from build123d import *

# Parameters (mm, degrees)
ESBO_O1_W                 = 105
ESBO_O1_H                 = 60
RESSALTO_EXTRUS_O1_DEPTH  = 1.7
ESBO_O2_W                 = 60
ESBO_O2_H                 = 15
ESBO_O2_W_2               = 40
RESSALTO_EXTRUS_O2_DEPTH  = 13.6
RESSALTO_EXTRUS_O6_START  = 11.6
ESBO_O3_W                 = 100
ESBO_O3_H                 = 53
RESSALTO_EXTRUS_O6_DEPTH  = 1.5
ESBO_O4_W                 = 62.184169383
ESBO_O4_H                 = 2.54
ESBO_O4_W_2               = 5.08
ESBO_O4_H_2               = 42.957805244
ESBO_O4_W_3               = 56.07185462
RESSALTO_EXTRUS_O8_DEPTH  = 11.6
ESBO_O6_W                 = 21
ESBO_O6_H                 = 22
RESSALTO_EXTRUS_O9_DEPTH  = 16
ESBO_O7_W                 = 25.746964405
ESBO_O7_H                 = 12
RESSALTO_EXTRUS_O10_DEPTH = 10
ESBO_O8_R                 = 1.5
CORTE_EXTRUS_O1_DEPTH     = 31.8
RESSALTO_EXTRUS_O11_DEPTH = 56.905179
CORTE_EXTRUS_O2_DEPTH     = 11
RESSALTO_EXTRUS_O12_START = 1
ESBO_O12_W                = 7
ESBO_O12_H                = 7
RESSALTO_EXTRUS_O12_DEPTH = 4


with BuildPart() as part:
    # Esbo_o1 → Ressalto-extrus_o1 (new body)
    with BuildSketch(Plane.XY):
        Rectangle(ESBO_O1_W, ESBO_O1_H)
    extrude(amount=RESSALTO_EXTRUS_O1_DEPTH)

    # Esbo_o2 → Ressalto-extrus_o2 (add)
    with BuildSketch(Plane.XY.offset(1.7)):
        with Locations((13.2, -12.2)):
            Rectangle(ESBO_O2_W, ESBO_O2_H)
        with Locations((3.2, 10.2)):
            Rectangle(ESBO_O2_W_2, ESBO_O2_H)
    extrude(amount=RESSALTO_EXTRUS_O2_DEPTH)



with BuildPart() as body_2:
    # Esbo_o3 → Ressalto-extrus_o6 (new body)
    with BuildSketch(Plane(origin=(0, 0, 0), x_dir=(-1, 0, 0), z_dir=(0, 0, -1)).offset(RESSALTO_EXTRUS_O6_START)):
        with Locations((2.5, 4.4)):
            Rectangle(ESBO_O3_W, ESBO_O3_H)
    extrude(amount=RESSALTO_EXTRUS_O6_DEPTH)


with BuildPart() as part_1:
    add(part.part)

    add(body_2.part)  # Ressalto-extrus_o8 merges body 2
    # Esbo_o4 → Ressalto-extrus_o8 (add)
    with BuildSketch(Plane.XY.offset(-11.6)):
        with Locations((7.150543675, 26.719832293)):
            Rectangle(ESBO_O4_W, ESBO_O4_H)
        with Locations((45.784919315, 5.42627648)):
            Rectangle(ESBO_O4_W_2, ESBO_O4_H_2)
        with Locations((10.206701056, -18.689881399)):
            Rectangle(ESBO_O4_W_3, ESBO_O4_H)
    extrude(amount=RESSALTO_EXTRUS_O8_DEPTH)

    # Esbo_o6 → Ressalto-extrus_o9 (add)
    with BuildSketch(Plane.XY.offset(1.7)):
        with Locations((-54, -9.6)):
            Rectangle(ESBO_O6_W, ESBO_O6_H)
    extrude(amount=RESSALTO_EXTRUS_O9_DEPTH)

    # Esbo_o7 → Ressalto-extrus_o10 (add)
    with BuildSketch(Plane.XY.offset(-11.6)):
        with Locations((-47.626517798, 17.9)):
            Rectangle(ESBO_O7_W, ESBO_O7_H)
    extrude(amount=RESSALTO_EXTRUS_O10_DEPTH)

    # Esbo_o8 → Corte-extrus_o1 (cut, through all)
    with BuildSketch(Plane(origin=(0, 0, -13.1), x_dir=(-1, 0, 0), z_dir=(0, 0, -1))):
        with Locations((37.26, 28.47)):
            Circle(ESBO_O8_R)
        with Locations((38.5, -19.7)):
            Circle(ESBO_O8_R)
        with Locations((-43.8, -19.7)):
            Circle(ESBO_O8_R)
    extrude(amount=-CORTE_EXTRUS_O1_DEPTH, mode=Mode.SUBTRACT)

    # Esbo_o9 → Ressalto-extrus_o11 (add)
    with BuildSketch(Plane.XZ.offset(30)):
        Polygon((49.5, 1.7), (49.5, 10.2), (58, 10.2), (58, 28.2), (49.5, 28.2), (49.5, 12.2), (47, 12.2), (47, 1.7), align=None)
    extrude(amount=-RESSALTO_EXTRUS_O11_DEPTH)

    # Esbo_o10 → Corte-extrus_o2 (cut)
    with BuildSketch(Plane(origin=(58, 0, 0), x_dir=(0, 0, -1), z_dir=(1, 0, 0))):
        Polygon((-10.2, -16.57372352), (-28.2, -16.57372352), (-28.2, -30), (-1.7, -30), (-1.7, -16.57372352), align=None)
    extrude(amount=-CORTE_EXTRUS_O2_DEPTH, mode=Mode.SUBTRACT)

    # Esbo_o12 → Ressalto-extrus_o12 (add)
    with BuildSketch(Plane.XZ.offset(30).offset(RESSALTO_EXTRUS_O12_START)):
        with Locations((-17, 5.2)):
            Rectangle(ESBO_O12_W, ESBO_O12_H)
    extrude(amount=-RESSALTO_EXTRUS_O12_DEPTH)


solid = part_1.part
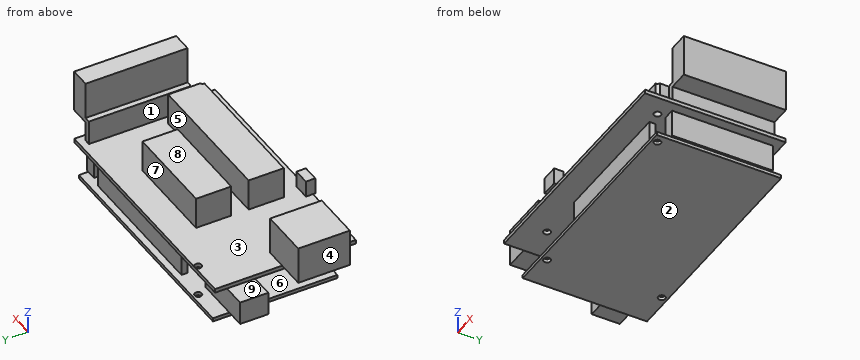
Model file for the job. Use its own axes, mm. Face numbers are marked on the shaded views. A direction names the side the tool comes from. Give positions to 0.01 mm unless a question says otherwise; leave off trailing zeros. Loops run counter-clockwise (first coordinate to the right, second up) from the corner with the lowest first, then second, coordinate; pieces in that order, holes last.
1) Pull direction X, two halves, no side cores. Call the marked faces 1, 2, 3 and 4: +X half, -X half, draft (parallel to the pull), parting line (faces both ways), or undercut.
2) Tool access for the marked faces 5, 6, 7, 8 and 9: list every direction of +Z, -Z, +X, -X, +Y, -Y with a clear straight run to the whole face (end or side of a thin tool).
3) Saw through at D-D (z = 3.5). Write the cut outline in (x, y).
4) Saw through at C-C (y = -13.5). Write the cut outline in (x, z), plus the area to 3 significant figures.
5) Saw through at A-A (x = -8.5). Write the cut outline in (y, z).
6) Saw through at B-B (x = -57). Write the cut outline in (y, z), plus the area to 3 significant figures.
7) Flat gauge pins, fed straight in: pin 1 Ø5 at (x, z) = (-50, -6) entering from +Y; pin 2 Ø16 at (x, y) = (-18, 10.5) entering from +Z; pin 3 Ø2 at (y, z) = (26.5, -7) entering from -X. Where does each tip first touch, or does it go through?
8) Wall check: line 1 (Z direction, x = -29, y = 13); line 2 (X direction, y = 0, z = 14.5); line 3 (Y direction, x = -38.5, z = 0.9). Give the ranges that are in metal, low to high.
Answer block:
1. face 1: undercut
1. face 2: draft
1. face 3: undercut
1. face 4: -X half
2. face 5: +Z
2. face 6: none
2. face 7: +Z, -X, +Y
2. face 8: +Z, -X, +Y, -Y
2. face 9: -X, +Y, -Y
3. outline: (-64.5, -20.6) - (-43.5, -20.6) - (-43.5, 1.4) - (-64.5, 1.4) - close; (-20.5, -31) - (-13.5, -31) - (-13.5, -27) - (-20.5, -27) - close; (-16.8, -19.7) - (42.3, -19.7) arc R1.5 cw to (43.2, -18.33) - (43.2, -4.7) - (-16.8, -4.7) - close; (-16.8, 2.7) - (23.2, 2.7) - (23.2, 17.7) - (-16.8, 17.7) - close; (47, -16.57) - (49.5, -16.57) - (49.5, 26.91) - (47, 26.91) - close
4. outline: (-64.5, 1.7) - (-52.5, 1.7) - (-52.5, 0) - (43.24, 0) - (43.24, -11.6) - (-52.5, -11.6) - (-52.5, -13.1) - (47.5, -13.1) - (47.5, -11.6) - (48.32, -11.6) - (48.32, 0) - (52.5, 0) - (52.5, 1.7) - (49.5, 1.7) - (49.5, 10.2) - (58, 10.2) - (58, 28.2) - (49.5, 28.2) - (49.5, 12.2) - (47, 12.2) - (47, 1.7) - (43.2, 1.7) - (43.2, 15.3) - (-16.8, 15.3) - (-16.8, 1.7) - (-43.5, 1.7) - (-43.5, 17.7) - (-64.5, 17.7) - close
4. area: 1,720 mm2
5. outline: (-30, 0) - (-19.96, 0) - (-19.96, -11.6) - (-22.1, -11.6) - (-22.1, -13.1) - (30.9, -13.1) - (30.9, -11.6) - (27.99, -11.6) - (27.99, 0) - (30, 0) - (30, 1.7) - (17.7, 1.7) - (17.7, 15.3) - (2.7, 15.3) - (2.7, 1.7) - (-4.7, 1.7) - (-4.7, 15.3) - (-19.7, 15.3) - (-19.7, 1.7) - (-30, 1.7) - close; hole (-17.42, -11.6) - (25.45, -11.6) - (25.45, 0) - (-17.42, 0) - close
6. outline: (-20.6, 1.7) - (1.4, 1.7) - (1.4, 17.7) - (-20.6, 17.7) - close; (11.9, -11.6) - (23.9, -11.6) - (23.9, -1.6) - (11.9, -1.6) - close
6. area: 472 mm2
7. pin 1: stops at y = 23.9
7. pin 2: stops at z = 15.3
7. pin 3: stops at x = -23.94
8. line 1: z = -13.1 to -11.6, 0 to 1.7
8. line 2: x = -64.5 to -43.5, 49.5 to 58
8. line 3: y = -30 to -21.2, -18.2 to 27.63, 29.31 to 30
